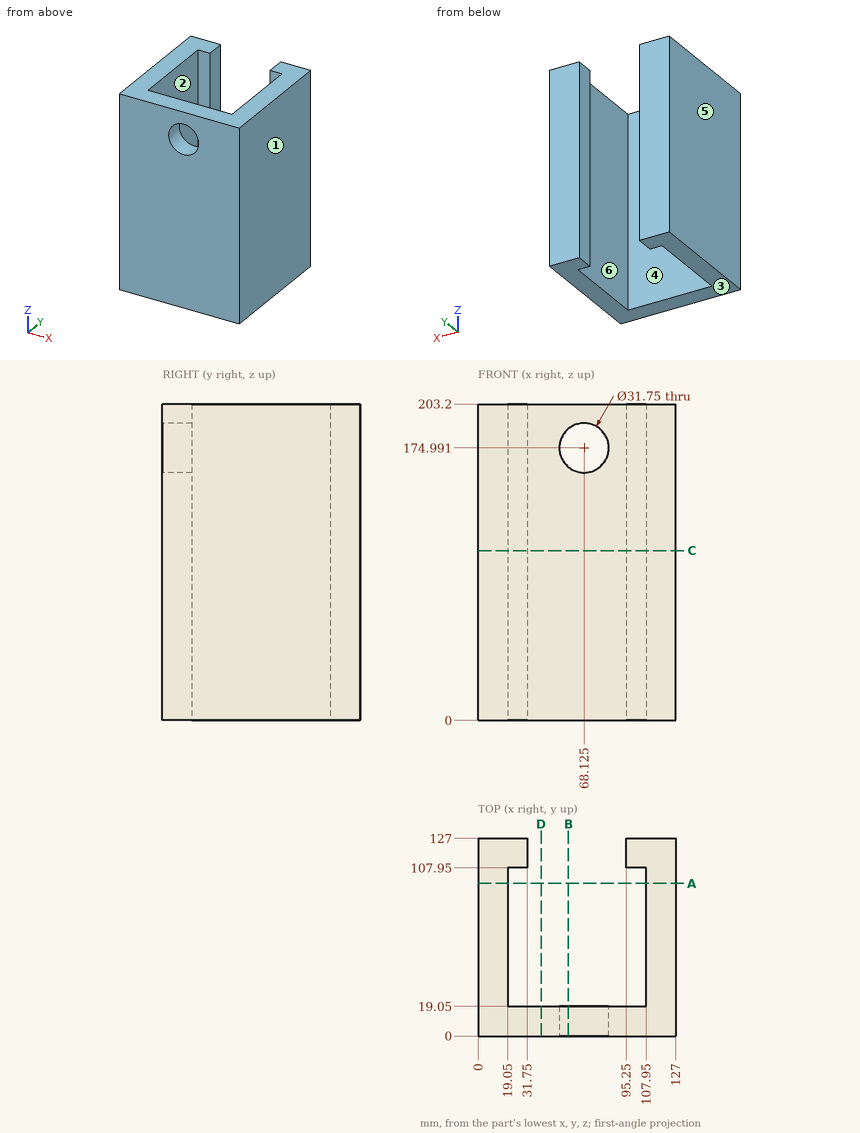
The drawing under review shows one solid part. Ordinate dimensions are in mm from its lowest x, y, z. A direction names the side the tool comes from. Coordinates: 2 decimals unless noted, no trailing zeros. Write each loop counter-clockwise with the first axis right and the second up, starting at its lowest first coordinate (ties: lowest second). Pieces come first, ordered by that corner, then holes. Notation, with made-up numbers: M -10.75,-20 L 2.25,-20 A29 ccw 2.25,4 Z; hole C 17.5,-9 d2. An arc over 180 degrees is marked long. Answer as a JSON object with one key per item and string values.
Item 1: Wall thickness on probe 1 along Y at (x, z) = (106, 156.5); probe 2 along Y at (x, z) = (73, 51): over which ranges is each line inside the solid? List them lowest first.
Outcome:
{"probe 1": "0 to 19.05, 107.95 to 127", "probe 2": "0 to 19.05"}
Item 2: Add section D-D, the plane x = 40.5. Give the boundary of the cut face in (y, z).
Outcome:
{"outline": "M 0,0 L 19.05,0 L 19.05,203.2 L 0,203.2 Z"}
Item 3: Insertion check: pin 1 Ø1.5 at (x, z) = (92, 133) entering from +Y. The pin has a flat end and moves straight along its axis. Give the tip position at first contact, or say it passes through.
Outcome:
{"pin 1": "y = 19.05"}
Item 4: Add section C-C, the plane z = 109. Give the boundary of the cut face in (x, y), and give its area (3 significant figures).
Outcome:
{"outline": "M 0,0 L 127,0 L 127,127 L 95.25,127 L 95.25,107.95 L 107.95,107.95 L 107.95,19.05 L 19.05,19.05 L 19.05,107.95 L 31.75,107.95 L 31.75,127 L 0,127 Z", "area": "7,020 mm²"}
Item 5: Add section B-B, the plane x = 58. Give the boundary of the cut face in (y, z), and give its area (4 significant figures).
Outcome:
{"outline": "M 0,0 L 19.05,0 L 19.05,162.76 L 0,162.76 Z; M 0,187.22 L 19.05,187.22 L 19.05,203.2 L 0,203.2 Z", "area": "3,405 mm²"}
Item 6: Add section A-A, the plane y = 98. Give the boundary of the cut face in (x, z), and give its area (3 significant figures).
Outcome:
{"outline": "M 0,0 L 19.05,0 L 19.05,203.2 L 0,203.2 Z; M 107.95,0 L 127,0 L 127,203.2 L 107.95,203.2 Z", "area": "7,740 mm²"}
Item 7: Machinability: for the marked faces 5 and 6, which of the approach directions +Z, -Z, +X, -X, +Y, -Y give a long, thin tool a straight path to every point of the face, cutting with its end or side? Answer none if there is none.
Outcome:
{"face 5": "+Z, -Z, -X, +Y, -Y", "face 6": "+Z, -Z"}
Item 8: Draft analysis for pull direction X (two halves, no side actions). For the marked faces 1, 2, 3 and 4, state which applies: pulls with the +X half, pulls with the -X half, needs draft (parallel to the pull), parting line crosses it, or undercut.
Outcome:
{"face 1": "pulls with the +X half", "face 2": "undercut", "face 3": "needs draft", "face 4": "undercut"}
